Work out the finished part from the listing and answer in its coordinate system (mm). A direction names the side the tool comes from. Coordinates: 2 decimals unless noted, no trailing zeros. Order: outer loops, then holes, each group sorted by start corner. A loop starts at its lowest first (then second) coordinate and runs counter-clockwise, first axis right, second up. Notation, with made-up numbers: (-24, 18.5) -> (23, 18.5) arc R24 ccw to (23, 54.5) -> close; hole circle Ø4 at (-17, 69). An arc over 180 degrees is marked (long way). Write item = value, one per line. Start each with the question number.
Q1. For a pull along Z with two mould halves and no side action, classify faces 1 (the flat face through (524, -7, -15.875)), 2 (the flat face through (82, -19, 146.05)), 3 (the flat face through (60.325, 451, -8)) as +Z half, -Z half, draft (parallel to the pull), parting line (faces both ways), or undercut.
Q2. The part is cut by section A-A, the plane z = 63.5. Determine the outline of the cut face in (x, y).
Q3. The part is cut by section B-B, the plane y = 262. Determine the outline of the cut face in (x, z) (3 decimals), plus the area to 3 significant figures.
Q4. Flat-ended cylindrical pins translate along their axes: pin 1 (10 mm diameter, centred on x = 358, z = 89.5, fed in from +Y); pin 2 (12.5 mm diameter, centred on y = -16.5, z = -4.5, fed in from -X) (3 decimals); pin 3 (1 mm diameter, centred on x = 556.5, y = 387, fed in from +Z) (3 decimals). Find the tip coordinate at first contact, or state that the pin passes through.
Q5. Which of the six approach directions +Z, -Z, +X, -X, +Y, -Y give full straight-line access (tool end or side, diameter ignored) to faces 4 (the flat face through (524, -31.75, -8)), 5 (the flat face through (583, 220, 10.16)), 6 (the flat face through (76, -13, 0)), 7 (the cylindrical face through (645.124, 109.736, 23.038)), 8 (the flat face through (76, 19.05, -8))?
Q6. The part is cut by section D-D, the plane y = 373. Determine the outline of the cut face in (x, z) (3 decimals), plus the area to 3 significant figures.
Q7. Straight lines are drawn through the part: L1, parallel to X at y = -19.05, z = -4 (3 decimals); L2, parallel to Y at x = 76.2, z = -12 (3 decimals); L3, parallel to Z at x = 491.5, y = 278.5 (3 decimals). For each, find the intervals that lie inside material, in ascending order. Write a range as from..to.
Q8. The part is cut by section C-C, the plane z = 190. Determine the outline of the cut face in (x, y).
```python
from build123d import *

# Parameters (mm, degrees)
F0_W      = 508
F0_H      = 444.5
F1_DEPTH  = 282.575
F2_W      = 31.75
F2_H      = 50.8
F2_W_2    = 50.8
F3_DEPTH  = 15.875
F4_W      = 723.9
F4_H      = 546.1
F5_DEPTH  = 38.1
F7_W      = 12.7
F7_H      = 266.7
F8_DEPTH  = 25.4
F9_W      = 38.1
F9_H      = 596.9
F10_DEPTH = 57.15
F11_W     = 254
F11_H     = 25.4
F12_DEPTH = 152.4
F13_R     = 50.8
F15_DEPTH = 25.4
F17_R     = 76.2
F18_DEPTH = 31.75
F20_R     = 76.2
F21_DEPTH = 31.75
F22_R     = 3.175
F23_DEPTH = 25.4
F24_R     = 19.05
F25_DEPTH = 25.4
F26_R     = 50.8
F27_DEPTH = 25.4
F28_R     = 15.875
F29_DEPTH = 50.8
F30_W     = 88.9
F30_H     = 114.3
F31_DEPTH = 38.1


with BuildPart() as f1:
    # F0 (on Top) → F1 (new body)
    with BuildSketch(Plane.XY):
        with Locations((254, 222.25)):
            Rectangle(F0_W, F0_H)
    extrude(amount=F1_DEPTH)

    # F2 (on face) → F3 (join)
    with BuildSketch(Plane(origin=(0, 0, 0), x_dir=(1, 0, 0), z_dir=(0, 0, -1))):
        with Locations((76.2, 6.35)):
            Rectangle(F2_W, F2_H)
        with Locations((523.875, 6.35)):
            Rectangle(F2_W_2, F2_H)
        with Locations((76.2, -450.85)):
            Rectangle(F2_W, F2_H)
        with Locations((523.875, -450.85)):
            Rectangle(F2_W_2, F2_H)
    extrude(amount=F3_DEPTH)

    # F4 (on face) → F5 (join)
    with BuildSketch(Plane.XY.offset(282.575)):
        with Locations((336.55, 196.85)):
            Rectangle(F4_W, F4_H)
    extrude(amount=F5_DEPTH)

    # F7 (on face) → F8 (cut)
    with BuildSketch(Plane.XY.offset(320.675)):
        with Locations((276.225, 222.25)):
            Rectangle(F7_W, F7_H)
    extrude(amount=-F8_DEPTH, mode=Mode.SUBTRACT)

    # F9 (on face) → F10 (join)
    with BuildSketch(Plane.XY.offset(320.675)):
        with Locations((425.7404655218, 171.45)):
            Rectangle(F9_W, F9_H)
    extrude(amount=F10_DEPTH)

    # F11 (on face) → F12 (join)
    with BuildSketch(Plane.YZ.offset(508)):
        with Locations((222.25, 22.86)):
            Rectangle(F11_W, F11_H)
    extrude(amount=F12_DEPTH)

    # F13
    f13_edges = [f1.edges().sort_by_distance(p)[0] for p in [
        (660.4, 95.25, 22.86),
        (660.4, 349.25, 22.86),
    ]]
    fillet(f13_edges, radius=F13_R)

    # F14 (on face) → F15 (join)
    with BuildSketch(Plane.XY.offset(320.675)):
        with BuildLine():
            ThreePointArc((-57.15, 31.75), (-47.8506403027, 9.2993596973), (-25.4, 0))
            Line((-25.4, 0), (-25.4, 95.25))
            ThreePointArc((-25.4, 95.25), (-47.8506403027, 85.9506403027), (-57.15, 63.5))
            Line((-57.15, 63.5), (-57.15, 31.75))
        make_face()
        with BuildLine():
            Line((-25.4, 330.2), (-25.4, 425.45))
            ThreePointArc((-25.4, 425.45), (-47.8506403027, 416.1506403027), (-57.15, 393.7))
            Line((-57.15, 393.7), (-57.15, 361.95))
            ThreePointArc((-57.15, 361.95), (-47.8506403027, 339.4993596973), (-25.4, 330.2))
        make_face()
    extrude(amount=-F15_DEPTH)

    # F17 (on offset) → F18 (join)
    with BuildSketch(Plane.XZ.offset(-57.15)):
        with Locations((12.7, 63.5)):
            Circle(F17_R)
    extrude(amount=-F18_DEPTH)

    # F20 (on offset) → F21 (join)
    with BuildSketch(Plane(origin=(0, 387.35, 0), x_dir=(-1, 0, 0), z_dir=(0, 1, 0))):
        with Locations((-12.7, 63.5)):
            Circle(F20_R)
    extrude(amount=-F21_DEPTH)

    # F22 (on face) → F23 (cut)
    with BuildSketch(Plane(origin=(0, 0, -15.875), x_dir=(1, 0, 0), z_dir=(0, 0, -1))):
        with Locations((76.2, 19.05)):
            Circle(F22_R)
        with Locations((76.2, -463.55)):
            Circle(F22_R)
        with Locations((527.05, -463.55)):
            Circle(F22_R)
        with Locations((527.05, 19.05)):
            Circle(F22_R)
    extrude(amount=-F23_DEPTH, mode=Mode.SUBTRACT)

    # F24 (on face) → F25 (join)
    with BuildSketch(Plane.XZ):
        with Locations((225.552, 152.4)):
            Circle(F24_R)
    extrude(amount=F25_DEPTH)

    # F26 (on face) → F27 (join)
    with BuildSketch(Plane.XZ.offset(25.4)):
        with Locations((225.552, 152.4)):
            Circle(F26_R)
    extrude(amount=F27_DEPTH)

    # F28 (on face) → F29 (join)
    with BuildSketch(Plane.XZ.offset(50.8)):
        with Locations((271.2737321854, 156.2635451555)):
            Circle(F28_R)
    extrude(amount=F29_DEPTH)

    # F30 (on face) → F31 (join)
    with BuildSketch(Plane.XZ):
        with Locations((82.55, 203.2)):
            Rectangle(F30_W, F30_H)
    extrude(amount=F31_DEPTH)


solid = f1.part
```
Model answer:
q1.face_1 = -Z half
q1.face_2 = undercut
q1.face_3 = draft
q2.outline = (-63.5, 57.15) -> (0, 57.15) -> (0, 0) -> (508, 0) -> (508, 444.5) -> (0, 444.5) -> (0, 387.35) -> (-63.5, 387.35) -> (-63.5, 355.6) -> (0, 355.6) -> (0, 88.9) -> (-63.5, 88.9) -> close
q3.outline = (-25.4, 282.575) -> (0, 282.575) -> (0, 0) -> (508, 0) -> (508, 10.16) -> (660.4, 10.16) -> (660.4, 35.56) -> (508, 35.56) -> (508, 282.575) -> (698.5, 282.575) -> (698.5, 320.675) -> (444.79, 320.675) -> (444.79, 377.825) -> (406.69, 377.825) -> (406.69, 320.675) -> (282.575, 320.675) -> (282.575, 295.275) -> (269.875, 295.275) -> (269.875, 320.675) -> (-25.4, 320.675) -> close
q3.area = 177,000 mm2
q4.pin_1 = 444.5
q4.pin_2 = 60.325
q4.pin_3 = 320.675
q5.face_4 = -Z, +X, -X, -Y
q5.face_5 = -Z, +X, +Y, -Y
q5.face_6 = +X, -X, -Y
q5.face_7 = -Z, +X, -Y
q5.face_8 = -Z, +X, -X
q6.outline = (-57.15, 295.275) -> (-25.4, 295.275) -> (-25.4, 282.575) -> (0, 282.575) -> (0, 138.634) arc R76.2 ccw (long way) to (54.821, 0) -> (508, 0) -> (508, 282.575) -> (698.5, 282.575) -> (698.5, 320.675) -> (444.79, 320.675) -> (444.79, 377.825) -> (406.69, 377.825) -> (406.69, 320.675) -> (-57.15, 320.675) -> close
q6.area = 182,000 mm2
q7.L1 = 60.325..73.025, 79.375..92.075, 498.475..523.875, 530.225..549.275
q7.L2 = -31.75..-22.225, -15.875..19.05, 425.45..460.375, 466.725..476.25
q7.L3 = 0..320.675
q8.outline = (0, 0) -> (38.1, 0) -> (38.1, -38.1) -> (127, -38.1) -> (127, 0) -> (508, 0) -> (508, 444.5) -> (0, 444.5) -> close; (191.39, -50.8) -> (259.71, -50.8) -> (259.71, -25.4) -> (191.39, -25.4) -> close
